Autodesk Inventor part; units mm, degrees
ref_plane "Work Plane1" through (52.1094, 0, 0) normal (0, 0, -1) x (-1, 0, 0)
ref_plane "YZ Plane" through (0, 0, 0) normal (1, 0, 0) x (0, 1, 0)
ref_plane "XZ Plane" through (0, 0, 0) normal (0, 1, 0) x (-1, 0, 0)
sketch "Schizzo1" plane through (0, 0, 0) normal (0, 0, 1) x (1, 0, 0)
  line L0 (-4.1484, 0) -> (22.0414, 0)
  line L1 (6.3771, 12) -> (4.5751, 15.8643)
  line L2 (6.3771, 12) -> (18.3, 12) construction
  line L3 (18.3, 12) -> (18.3, 0) construction
  arc A0 (4.5751, 15.8643) -> (0, 14.85) centre (2.4, 14.85) ccw
  line L4 (6.3771, 12) -> (6.3771, 0)
  line L5 (0, -3.5401) -> (0, 21.2403)
  point P0 (0, 0)
  dimension "d1" = 24
  dimension "d3" = 34.5
  dimension "d4" = 2.4
  dimension "d16" = 18.3
  dimension "d17" = 25
revolve "Anello" add sketch "Schizzo1" angle 360 about axis through (-10, 0, 0) along (1, 0, 0)
sketch "Schizzo2" plane through (0, 0, 0) normal (-1, 0, 0) x (0, 0, 1)
  circle A0 centre (0, 0) radius 4.9
  line L0 (-12, -6.9282) -> (-12, 6.9282)
  line L1 (-12, 6.9282) -> (0, 13.8564)
  line L2 (0, 13.8564) -> (12, 6.9282)
  line L3 (12, 6.9282) -> (12, -6.9282)
  line L4 (12, -6.9282) -> (0, -13.8564)
  line L5 (0, -13.8564) -> (-12, -6.9282)
  circle A1 centre (0, 0) radius 14.85
  dimension "d5" = 27.7128
extrude "Corpo" add sketch "Schizzo2" against normal blind 15.3 contours A0 | L0 L1 L2 L3 L4 L5
sketch "Schizzo3" plane through (15.3, 0, 0) normal (1, 0, 0) x (0, 0, -1)
  circle A0 centre (0, 0) radius 12
  dimension "d19" = 24
extrude "Corona" add sketch "Schizzo3" along normal blind 3
sketch "Schizzo4" plane through (0, 0, 0) normal (-1, 0, 0) x (0, 0, 1)
  circle A0 centre (0, 0) radius 4.9
  circle A1 centre (0, 0) radius 14.85
hole "Filettatura" at (0, 0, 0) direction (1, 0, 0) diameter 13.835 end through all
sketch "Schizzo5" plane through (0, 0, 0) normal (0, 0, 1) x (1, 0, 0)
  line L0 (5.5114, 13.8564) -> (15.3, 13.8564)
  line L1 (15.3, 6.9282) -> (15.3, 13.8564)
  line L2 (0, -14.85) -> (0, 14.85)
  line L3 (-3.06, 0) -> (18.36, 0)
  line L4 (14.2282, 13.8564) -> (15.3, 12)
  dimension "d9" = 30
  dimension "d10" = 24
revolve "Smusso1" cut sketch "Schizzo5" angle 360 about axis through (-10, 0, 0) along (1, 0, 0)
chamfer "Smusso2" distance 1.0825 angle 30 1 edges at (0, 0, -6.9175) measured on face at (0, 12.0452, -1.4626)
ref_plane "Work Plane1" through (52.1094, 0, 0) normal (0, 0, -1) x (-1, 0, 0)
equation "\"d1\" = SW"
equation "\"d3\" = LADI"
equation "\"d4\" = PHH"
equation "\"d16\" = KOH"
equation "\"d17\" = KEWI"
equation "\"d5\" = 1.1547 * SW"
equation "\"d6\" = KOH1"
equation "\"d19\" = SD2"
equation "\"d11\" = KOH - KOH1"
equation "\"d9\" = ANG1"
equation "\"d10\" = SW0"
equation "\"d13\" = -0.5 * GD1 + 0.5 * NND"
equation "\"d57\" = -0.5 * GD1 + 0.5 * NND"
equation "\"ANG1\" = 30deg"
equation "\"KEWI\" = 25deg"
equation "\"NND\" = 16"
equation "\"LADI\" = 34.5"
equation "\"SW\" = 24"
equation "\"PHH\" = 2.4"
equation "\"KOH\" = 18.3"
equation "\"SW0\" = SW"
equation "\"d0\" = LADI"
equation "\"d2\" = PHH"
equation "\"KOH1\" = 15.3"
equation "\"SD2\" = SW"
equation "\"GUL\" = 0.541266 * PTC"
equation "\"RR\" = PHH"
equation "\"THREADDIA\" = 16"
equation "\"TOA\" = 30deg"
equation "\"PTC\" = 2"
equation "\"GAL\" = 0.541266 * PTC"
equation "\"E0\" = 1.155 * SW"
equation "\"PG\" = 1.2345"
equation "\"Mw\" = 8.9"
equation "\"r\" = 1"
properties part number "ISO 7044 - M16" material "Acciaio"
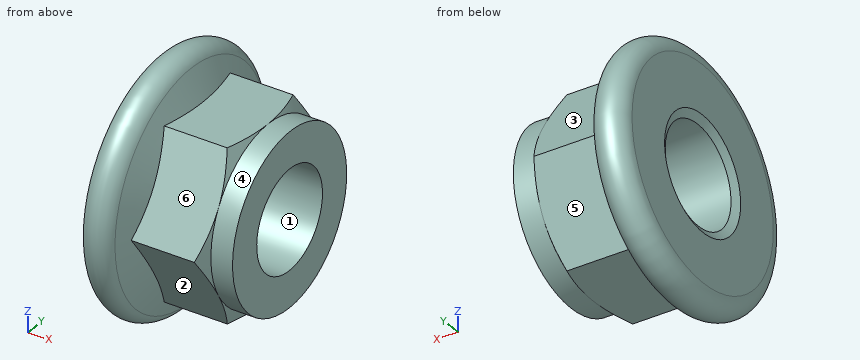
Read the model definition and answer for the solid it produces. Units are mm, in the model's axes. Face numbers are marked on the shaded views. A direction names the side the tool comes from. Give positions to 0.01 mm unless a question says otherwise; leave off trailing zeros. Order: outer loops, then holes, each group sorted by start corner. A loop starts at its lowest first (then second) coordinate and runs counter-clockwise, first axis right, second up. Notation, with made-up numbers: (10, 11) -> (34, 11) arc R24 ccw to (34, 49) -> close; hole circle Ø9 at (40, 9.25). An arc over 180 degrees is marked (long way). One line per item, written item: value. Start each with the question number.
(1) The part is cut by section B-B (x = 2). Determine the outline of the cut face in (y, z) (1 decimal), and give its area (3 significant figures).
(2) For a pull along Z with two mould halves and no side action, classify the marked faces 1, 2 and 3 as released by +Z, released by -Z, zero draft, split by the parting line, or undercut.
(3) The part is cut by section A-A (x = 8.75). Determine the outline of the cut face in (y, z) (1 decimal), and give its area (4 significant figures).
(4) Flat-ended cylindrical pins translate along their axes: P1, Ø3, axis at y = -3.5, z = -2, coming from the +X side; P2, Ø6, axis at x = 4.5, z = -5, coming from the +Y side; P3, Ø4, axis at y = -13, z = 8.5, coming from the +X side; P4, Ø8, axis at x = 9, y = -3.5, coming from the +Z side. Find the tip coordinate at first contact, or state that the pin passes through.
(5) A tool of negligible diameter and unlimited length cuts with its end or side. For the marked faces 4, 5 and 6, from which of +Z, -Z, +X, -X, +Y, -Y can it reach the whole face along a straight path? Write none if from no direction.
(6) Straight lines are drawn through the part: L1, parallel to Z at x = 14.75, y = 0; L2, parallel to Y at x = 9, z = 0; L3, parallel to Z at x = 5.75, y = 0. For each, find the intervals that lie inside material, in ascending order.
Taken from the geometry:
1. outline: circle Ø34.4 at (0, 0); hole circle Ø13.8 at (0, 0)
1. area: 781 mm^2
2. face 1: undercut
2. face 2: released by -Z
2. face 3: released by +Z
3. outline: (-13.9, 0) -> (-6.9, -12) -> (6.9, -12) -> (13.9, 0) -> (6.9, 12) -> (-6.9, 12) -> close; hole circle Ø13.8 at (0, 0)
3. area: 348.5 mm^2
4. P1: through
4. P2: y = 17.03
4. P3: x = 5.66
4. P4: z = 14.58
5. face 4: +X
5. face 5: -Z, +X, +Y
5. face 6: +Z, +X, -Y
6. L1: -12 to -6.92, 6.92 to 12
6. L2: -13.86 to -6.92, 6.92 to 13.86
6. L3: -13.34 to -6.92, 6.92 to 13.34
